The listing builds one solid part. Answer for the finished solid, in the listing's coordinates (mm). Round coordinates to 2 decimals unless told otherwise and drop trailing zeros. Loops run counter-clockwise (first coordinate to the right, second up) from the corner with the lowest first, then second, coordinate; pieces in that order, holes last. Notation, with made-up numbers: M 27.25,69.25 L 31.25,69.25 A27 cw 31.25,89.25 Z; hole C 63.25,-7 d10. An arc over 180 degrees is marked long. Answer as a JSON object with one key per item and string values.
Autodesk Inventor part; units mm, degrees
ref_plane "YZ Plane" through (0, 0, 0) normal (1, 0, 0) x (0, 1, 0)
ref_plane "XZ Plane" through (0, 0, 0) normal (0, 1, 0) x (-1, 0, 0)
ref_plane "XY Plane" through (0, 0, 0) normal (0, 0, 1) x (1, 0, 0)
sketch "Sketch1" plane through (0, 0, 0) normal (0, 1, 0) x (-1, 0, 0)
  line L0 (3.175, -3.175) -> (22.225, -3.175)
  line L1 (0, 161.925) -> (0, 0)
  line L2 (25.4, 161.925) -> (25.4, 120.65)
  line L3 (50.8, 95.25) -> (95.25, 95.25)
  line L4 (25.4, 0) -> (25.4, 44.45)
  line L5 (50.8, 69.85) -> (95.25, 69.85)
  arc A0 (25.4, 120.65) -> (50.8, 95.25) centre (50.8, 120.65) ccw
  line L6 (0, 0) -> (3.175, -3.175)
  line L7 (25.4, 0) -> (22.225, -3.175)
  arc A1 (50.8, 69.85) -> (25.4, 44.45) centre (50.8, 44.45) ccw
  line L8 (98.425, 73.025) -> (98.425, 92.075)
  line L9 (98.425, 73.025) -> (95.25, 69.85)
  line L10 (95.25, 95.25) -> (98.425, 92.075)
  line L11 (25.4, 161.925) -> (25.4, 165.1)
  line L12 (0, 161.925) -> (0, 165.1)
  line L13 (0, 165.1) -> (0, 165.1)
  line L14 (3.175, 168.275) -> (22.225, 168.275)
  line L15 (25.4, 165.1) -> (25.4, 165.1)
  line L16 (22.225, 168.275) -> (25.4, 165.1)
  line L17 (3.175, 168.275) -> (0, 165.1)
  point P0 (92.075, 69.85)
  point P1 (95.25, 69.85)
  point P2 (0, 168.275)
  point P3 (25.4, 168.275)
  dimension "d6" = 25.4
  dimension "d21" = 25.4
  dimension "d44" = 165.1
  dimension "d63" = 44.45
  dimension "d64" = 44.45
  dimension "d65" = 3.175
  dimension "d67" = 3.175
  dimension "d70" = 3.175
  dimension "d91" = 3.175
  dimension "d92" = 3.175
  dimension "d93" = 3.175
  dimension "d94" = 3.175
extrude "Extrusion1" add sketch "Sketch1" along normal blind 2.54
hole "Hole2" at (-12.7, 2.54, 82.55) direction (0, -1, 0) diameter 6.35 end through all
pattern_linear "Rectangular Pattern4" count 4 spacing 25.4 along (-1, 0, 0) of "Hole2"
pattern_linear "Rectangular Pattern5" count 7 spacing 25.4 along (0, 0, -1) of "Hole2" first direction both ways yes
equation "\"d21\" = d6"
equation "\"d67\" = d65"
equation "\"d79\" = Thickness"
equation "\"BendRadius\" = Thickness"
equation "\"BendReliefWidth\" = Thickness"
equation "\"BendReliefDepth\" = 0.5 * Thickness"
equation "\"CornerReliefSize\" = 4 * Thickness"
equation "\"MinimumRemnant\" = 2 * Thickness"
equation "\"TransitionRadius\" = BendRadius"
equation "\"JacobiRadiusSize\" = BendRadius"
equation "\"GapSize\" = Thickness"
properties part number "T-gusset"
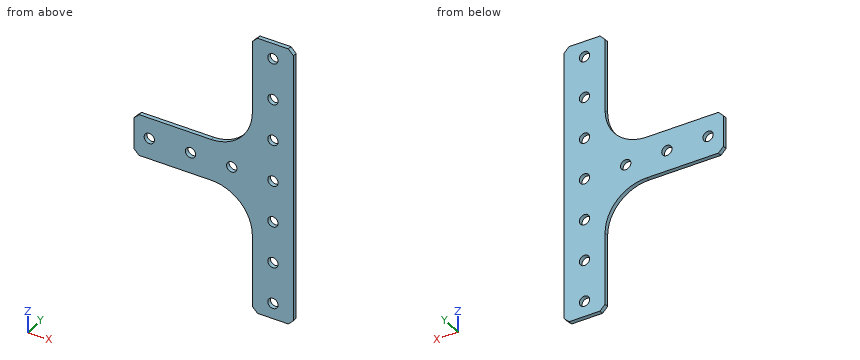
Item 1: The part is cut by section C-C (y = 1.5). Give the number of separate pieces and of enclosed holes in the cut face, then the cut area to 3 significant figures.
Values follow:
{"separate pieces": "1", "enclosed holes": "10", "area": "6,140 mm^2"}
Item 2: The part is cut by section A-A (x = -88.9). Give the vertices of the cut face in (y, z) (3 decimals).
Values follow:
{"outline": "M 0,69.85 L 2.54,69.85 L 2.54,79.375 L 0,79.375 Z; M 0,85.725 L 2.54,85.725 L 2.54,95.25 L 0,95.25 Z"}
Item 3: Straight lines are drawn through the part: line 1 (X direction, y = 1.85, z = 82.55) (3 decimals); line 2 (X direction, y = 2.3, z = 80) (3 decimals); line 3 (X direction, y = 1.7, z = 133.35) (3 decimals). For each, find the intervals that lie inside material, in ascending order.
Values follow:
{"line 1": "-98.425 to -92.075, -85.725 to -66.675, -60.325 to -41.275, -34.925 to -15.875, -9.525 to 0", "line 2": "-98.425 to -90.792, -87.008 to -65.392, -61.608 to -39.992, -36.208 to -14.592, -10.808 to 0", "line 3": "-25.4 to -15.875, -9.525 to 0"}
Item 4: Flat-ended cylindrical pins translate along their axes: P1, Ø1, axis at x = -85.5, y = 2, coming from the -Z side; P2, Ø5.5, axis at x = -38.1, z = 82.55, coming from the +Y side; P3, Ø1.3, axis at y = 1.5, z = 138.5, coming from the -X side. Find the tip coordinate at first contact, or state that the pin passes through.
Values follow:
{"P1": "z = 69.85", "P2": "through", "P3": "x = -25.4"}
Item 5: The part is cut by section D-D (z = 31.75). Give the vertices of the cut face in (x, y) (3 decimals), then the cut area to 3 significant figures.
Values follow:
{"outline": "M -25.4,0 L -15.875,0 L -15.875,2.54 L -25.4,2.54 Z; M -9.525,0 L 0,0 L 0,2.54 L -9.525,2.54 Z", "area": "48.4 mm^2"}
Item 6: The part is cut by section B-B (z = 82.55). Give the vertices of the cut face in (x, y) (3 decimals), then the cut area to 3 significant figures.
Values follow:
{"outline": "M -98.425,0 L -92.075,0 L -92.075,2.54 L -98.425,2.54 Z; M -85.725,0 L -66.675,0 L -66.675,2.54 L -85.725,2.54 Z; M -60.325,0 L -41.275,0 L -41.275,2.54 L -60.325,2.54 Z; M -34.925,0 L -15.875,0 L -15.875,2.54 L -34.925,2.54 Z; M -9.525,0 L 0,0 L 0,2.54 L -9.525,2.54 Z", "area": "185 mm^2"}
